Verification items for the finished model (mm, model axes). A direction names the side the tool comes from. Round coordinates to 2 decimals unless told otherwise and drop trailing zeros. Loops run counter-clockwise (first coordinate to the right, second up) from the corner with the lowest first, then second, coordinate; pieces in that order, holes last. Notation, with made-up numbers: (-4, 31) -> (47, 31) arc R19 ccw to (47, 35) -> close; hole circle Ø7 at (-32, 1.25). An arc over 180 degrees is marked (long way). Use a Markdown table: item, result. Add a question column.
Autodesk Inventor part; units mm, degrees
ref_plane "YZ Plane" through (0, 0, 0) normal (1, 0, 0) x (0, 1, 0)
ref_plane "XZ Plane" through (0, 0, 0) normal (0, 1, 0) x (-1, 0, 0)
ref_plane "XY Plane" through (0, 0, 0) normal (0, 0, 1) x (1, 0, 0)
sketch "스케치1" plane through (0, 0, 0) normal (0, 1, 0) x (-1, 0, 0)
  line L0 (-12.5, 16) -> (12.5, 16)
  line L1 (12.5, 16) -> (12.5, -16)
  line L2 (12.5, -16) -> (-12.5, -16)
  line L3 (-12.5, -16) -> (-12.5, 16)
  line L4 (-12.5, 16) -> (12.5, -16) construction
  line L5 (12.5, 16) -> (-12.5, -16) construction
  point P0 (0, 0)
  dimension "d0" = 25
  dimension "d1" = 32
extrude "돌출1" add sketch "스케치1" along normal blind 5
sketch "스케치2" plane through (0, 5, 0) normal (0, 1, 0) x (1, 0, 0)
  line L0 (-12.4719, -15.8) -> (12.5281, -15.8)
  line L1 (12.5281, -15.8) -> (12.5281, -10.8)
  line L2 (12.5281, -10.8) -> (-12.4719, -10.8)
  line L3 (-12.4719, -10.8) -> (-12.4719, -15.8)
  line L4 (-12.5, 16) -> (-12.5, -16)
  line L5 (-12.5, 0) -> (12.5281, 0)
  line L6 (-12.4719, 15.8) -> (12.5281, 15.8)
  line L7 (12.5281, 15.8) -> (12.5281, 10.8)
  line L8 (12.5281, 10.8) -> (-12.4719, 10.8)
  line L9 (-12.4719, 10.8) -> (-12.4719, 15.8)
  line L10 (-12.5, -16) -> (-12.5, 16)
  point P0 (0, 0)
  dimension "d4" = 25
  dimension "d5" = 5
  dimension "d24" = 21.6
extrude "돌출2" add sketch "스케치2" along normal blind 15
sketch "스케치3" plane through (12.5, 5, -15.8) normal (0, 0, -1) x (-1, 0, 0)
  circle A0 centre (7.4824, 7.5) radius 1.25
  line L0 (12.5, -5) -> (12.4719, 15)
  line L1 (24.9719, 15) -> (-0.0281, 15)
  line L2 (0, 0) -> (25, 0)
  circle A1 centre (17.4824, 7.514) radius 1.25
  dimension "d8" = 2.5
  dimension "d9" = 5
  dimension "d10" = 7.5
extrude "돌출3" cut sketch "스케치3" against normal up to surface (31.6 mm away)
sketch "스케치4" plane through (0, 0, 0) normal (0, -1, 0) x (1, 0, 0)
  line L0 (-12.5, -16) -> (-12.5, 16)
  line L1 (12.5, 10.8) -> (12.5, -10.8)
  line L2 (-12.5, 13) -> (12.5, 13)
  line L3 (12.5, 13) -> (12.5, 8)
  line L4 (12.5, 8) -> (-12.5, 8)
  line L5 (-12.5, 8) -> (-12.5, 13)
  line L6 (-12.5, 0) -> (12.5, 0)
  line L7 (-12.5, 16) -> (-12.5, -16)
  line L8 (12.5, -10.8) -> (12.5, 10.8)
  line L9 (-12.5, -13) -> (12.5, -13)
  line L10 (12.5, -13) -> (12.5, -8)
  line L11 (12.5, -8) -> (-12.5, -8)
  line L12 (-12.5, -8) -> (-12.5, -13)
  point P0 (0, 0)
  point P1 (12.5, -8)
  point P2 (-12.5, -13)
  dimension "d13" = 8
  dimension "d14" = 5
extrude "돌출4" add sketch "스케치4" along normal blind 10 contours L0 L11 L1 L10 L9 | L0 L2 L3 L1 L4
sketch "스케치5" plane through (12.5, 0, -13) normal (0, 0, -1) x (-1, 0, 0)
  circle A0 centre (17.5, -5) radius 1.25
  line L0 (25, -10) -> (0, -10)
  line L1 (25, 0) -> (25, -10)
  line L2 (12.5, -10) -> (12.5, 0)
  circle A1 centre (7.5, -5) radius 1.25
  dimension "d17" = 2.5
  dimension "d18" = 5
  dimension "d22" = 5
extrude "돌출5" cut sketch "스케치5" against normal up to surface (26 mm away)
properties part number "Tensile_test_bottom_adapter2"
1) Sectioned sample at B-B on x = 0.5. Enter the section's corners in (y, z).
2) Sectioned sample at C-C on z = -9. Enter the section's corners in (x, y).
3) Access from +Z, -Z, +X, -X, +Y, -Y to the whole of each face (thin tool, end or side, straight path). Record for faces 4 (the face through (0, 12, -15.8)), 5 (the face through (0, -5, 8)), 6 (the face through (0, -5, 13)), 7 (the face through (0, 12, -10.8)), 8 (the face through (0, -5, -13)).
4) Go/stop test with flat-tipped pins: pin 1 (11 mm diameter, centred on x = 6, y = -7.5, fed in from -Z); pin 2 (10 mm diameter, centred on x = 8.5, z = 2.5, fed in from +Y); pin 3 (4.5 mm diameter, centred on x = -0.5, y = 11, fed in from +Z). Record where each tip stops, or that it passes through.
5) Release check for a two-part mould opening along Y. For faces 1 (the face through (0, -5, -8)), 2 (the face through (5.27, -6.22, -10.54)), 3 (the face through (0, 0, 15)) record: released by +Y, released by -Y, zero draft, split by the parting line, or undercut.
6) Thickness scan on line 1 (Z direction, x = -6.5, y = 7.5); line 2 (Y direction, x = -5, z = -11.8); line 3 (Z direction, x = -10.75, y = -0.5). Record the ranges inside material, lowest first.
7) Sectioned sample at A-A on y = -5. Enter the section's corners in (x, z).
8) Sectioned sample at D-D on z = 6. Enter the section's corners in (x, y).
Geometry results:
| question | item | result |
|---|---|---|
| 1 | outline | (-10, -13) -> (0, -13) -> (0, -16) -> (5, -16) -> (5, -15.8) -> (20, -15.8) -> (20, -10.8) -> (5, -10.8) -> (5, 10.8) -> (20, 10.8) -> (20, 15.8) -> (5, 15.8) -> (5, 16) -> (0, 16) -> (0, 13) -> (-10, 13) -> (-10, 8) -> (0, 8) -> (0, -8) -> (-10, -8) -> close |
| 2 | outline | (-12.5, -10) -> (12.5, -10) -> (12.5, 5) -> (-12.5, 5) -> close; hole circle Ø2.5 at (-5, -5); hole circle Ø2.5 at (5, -5) |
| 3 | face 4 | -Z, +X, -X, +Y |
| 3 | face 5 | +X, -X, -Y |
| 3 | face 6 | +Z, +X, -X, -Y |
| 3 | face 7 | +X, -X, +Y |
| 3 | face 8 | -Z, +X, -X, -Y |
| 4 | pin 1 | z = -13 |
| 4 | pin 2 | y = 5 |
| 4 | pin 3 | z = 15.8 |
| 5 | face 1 | zero draft |
| 5 | face 2 | undercut |
| 5 | face 3 | released by -Y |
| 6 | line 1 | -15.8 to -10.8, 10.8 to 15.8 |
| 6 | line 2 | -10 to -6.25, -3.75 to 11.26, 13.76 to 20 |
| 6 | line 3 | -13 to -8, 8 to 13 |
| 7 | outline | (-12.5, -13) -> (-6.25, -13) -> (-6.25, -8) -> (-12.5, -8) -> close; (-12.5, 8) -> (-6.25, 8) -> (-6.25, 13) -> (-12.5, 13) -> close; (-3.75, -13) -> (3.75, -13) -> (3.75, -8) -> (-3.75, -8) -> close; (-3.75, 8) -> (3.75, 8) -> (3.75, 13) -> (-3.75, 13) -> close; (6.25, -13) -> (12.5, -13) -> (12.5, -8) -> (6.25, -8) -> close; (6.25, 8) -> (12.5, 8) -> (12.5, 13) -> (6.25, 13) -> close |
| 8 | outline | (-12.5, 0) -> (12.5, 0) -> (12.5, 5) -> (-12.5, 5) -> close |
